from build123d import *

# Parameters (mm, degrees)
SKETCH1_R           = 0.75
BOSS_EXTRUDE1_DEPTH = 4


with BuildPart() as part:
    # Sketch1 → Boss-Extrude1 (new body)
    with BuildSketch(Plane(origin=(0, 0, 0), x_dir=(0, 0, -1), z_dir=(1, 0, 0))):
        with BuildLine():
            Line((59.464274989, 10.5), (24.464274989, 10.5))
            ThreePointArc((24.464274989, 10.5), (7.885689727, 13.874194792), (-2.453052661, 0.482216385))
            ThreePointArc((-2.453052661, 0.482216385), (1.193550555, -2.19668775), (0.930226833, 2.320490905))
            ThreePointArc((0.930226833, 2.320490905), (11.73957945, 11.763813024), (24.654031937, 5.5))
            Line((24.654031937, 5.5), (59.464274989, 5.5))
            ThreePointArc((59.464274989, 5.5), (61.964274989, 8), (59.464274989, 10.5))
        make_face()
        with Locations((59.464274989, 8)):
            Circle(SKETCH1_R, mode=Mode.SUBTRACT)
        Circle(SKETCH1_R, mode=Mode.SUBTRACT)
    extrude(amount=BOSS_EXTRUDE1_DEPTH)


solid = part.part
Could you check a few things on this model? Use its own coordinates, in mm. A direction names the side the tool comes from. Give positions to 0.01 mm unless a question says otherwise; leave off trailing zeros. Write each loop counter-clockwise with the first axis right and the second up, starting at its lowest first coordinate (ties: lowest second). Pieces come first, ordered by that corner, then holes. Notation, with made-up numbers: (-22.5, 50) - (-6.5, 50) arc R13 ccw to (-6.5, 57) - close; hole circle Ø10 at (42, -19). An arc over 180 degrees is marked (long way). Use CSV: the item, a comma, the result in double quotes. Start each with the question number.
Item 1: If I drill on line 1 along Y through (x, z) = (2.85, -33); line 2 along Z through (x, y) = (1.1, 10); line 3 along Z through (x, y) = (0.8, 7.75), over which ranges is the centre line in solid material (lowest first)?
Item 2: For faces 1 (the face through (2, 5.5, -42)), 2 (the face through (2, 10.5, -42)), 3 (the face through (1.97, 0.03, 0.75)), which set-ups out of +Z, -Z, +X, -X, +Y, -Y let a thin tool reach every point of the face, with its end or its side?
Item 3: I'm going to push flat-ended pins straight in: pin 1 (1 mm diameter, centred on x = 2.5, y = 3, fed in from -Z); pin 2 (1.5 mm diameter, centred on x = 3, z = -44.5, fed in from -Y); pin 3 (1 mm diameter, centred on y = 9.5, z = -23, fed in from -X). Where does each tip first touch, or does it pass through?
Item 4: If we mould it in two halves opening along Y, with no side actions, what happens to faces 4 (the face through (0, 8, -30)), 5 (the face through (1.972, -2.233, -1.123)), 6 (the face through (1.97, 13.96, -8.12))? For each: pulls with the +Y half, pulls with the -Y half, needs draft (parallel to the pull), parting line crosses it, or undercut.
Item 5: I want a section at A-A, the plane x = 2.25. Please give me the cut outline in (y, z), then the cut area to 3 significant figures.
Item 6: I want a section at C-C, the plane z = 0. Please give me the cut outline in (x, y).
Item 7: I want a section at D-D, the plane z = -43.5. Please give me the cut outline in (x, y).
Item 8: I want a section at B-B, the plane y = 8. Please give me the cut outline in (x, z).
Findings:
1,line 1,"y = 5.5 to 10.5"
1,line 2,"z = -60.96 to -20.2, -6.73 to -1.96"
1,line 3,"z = -61.95 to -60.17, -58.76 to -22.97, -3.96 to -0.15"
2,face 1,"-Z, +X, -X, -Y"
2,face 2,"-Z, +X, -X, +Y"
2,face 3,"+X, -X"
3,pin 1,"stops at z = -1.32"
3,pin 2,"stops at y = 5.5"
3,pin 3,"stops at x = 0"
4,face 4,"needs draft"
4,face 5,"undercut"
4,face 6,"pulls with the +Y half"
5,outline,"(0.48, 2.45) arc R2.5 ccw (long way) to (2.32, -0.93) arc R13 cw to (5.5, -24.65) - (5.5, -59.46) arc R2.5 ccw to (10.5, -59.46) - (10.5, -24.46) arc R16 ccw to start; hole circle Ø1.5 at (0, 0); hole circle Ø1.5 at (8, -59.46)"
5,area,"297 mm2"
6,outline,"(0, -2.5) - (4, -2.5) - (4, -0.75) - (0, -0.75) - close; (0, 0.75) - (4, 0.75) - (4, 7.52) - (0, 7.52) - close"
7,outline,"(0, 5.5) - (4, 5.5) - (4, 10.5) - (0, 10.5) - close"
8,outline,"(0, -61.96) - (4, -61.96) - (4, -60.21) - (0, -60.21) - close; (0, -58.71) - (4, -58.71) - (4, -22.73) - (0, -22.73) - close; (0, -4.2) - (4, -4.2) - (4, -0.32) - (0, -0.32) - close"
